from build123d import *

# Parameters (mm, degrees)
SKETCH_1_W          = 6
SKETCH_1_H          = 4
EXTRUDE_1_DEPTH     = 2
EXTRUDE_2_DEPTH     = 2
EXTRUDE_3_DEPTH     = 2
CUT_EXTRUDE_1_DEPTH = 2
CUT_EXTRUDE_2_DEPTH = 2


with BuildPart() as part:
    # 草圖1 → 填料-伸長1 (new body)
    with BuildSketch(Plane(origin=(0, 0, 0), x_dir=(1, 0, 0), z_dir=(0, 1, 0))):
        with Locations((3, 2)):
            Rectangle(SKETCH_1_W, SKETCH_1_H)
    extrude(amount=EXTRUDE_1_DEPTH)

    # 草圖2 → 填料-伸長2 (add)
    with BuildSketch(Plane(origin=(0, 2, 0), x_dir=(1, 0, 0), z_dir=(0, 1, 0))):
        Polygon((0, 4), (6, 2), (6, 4), align=None)
    extrude(amount=EXTRUDE_2_DEPTH)

    # 草圖4 → 填料-伸長3 (add)
    with BuildSketch(Plane(origin=(0, 2, 0), x_dir=(1, 0, 0), z_dir=(0, 1, 0))):
        Polygon((0, 0), (0, 2), (6, 0), align=None)
    extrude(amount=EXTRUDE_3_DEPTH)

    # Sketch 3D_1 → 除料-伸長1 (cut, along a direction that is not the sketch's normal)
    with BuildSketch(Plane(origin=(6, 2, -4), x_dir=(-0.9486832980505139, 0.316227766016838, 0), z_dir=(0.2294157338705617, 0.6882472016116854, -0.6882472016116854))):
        Polygon((0, 0), (0.632455532, 2.75680975), (6.32455532, 0), align=None)
    extrude(amount=CUT_EXTRUDE_1_DEPTH, dir=(0, 1, 0), mode=Mode.SUBTRACT)

    # Sketch 3D_2 → 除料-伸長2 (cut, along a direction that is not the sketch's normal)
    with BuildSketch(Plane(origin=(0, 2, 0), x_dir=(0.9486832980505139, 0.316227766016838, 0), z_dir=(-0.22941573387056177, 0.6882472016116853, 0.6882472016116854))):
        Polygon((0, 0), (0.632455532, 2.75680975), (6.32455532, 0), align=None)
    extrude(amount=CUT_EXTRUDE_2_DEPTH, dir=(0, 0, 1), mode=Mode.SUBTRACT)


solid = part.part
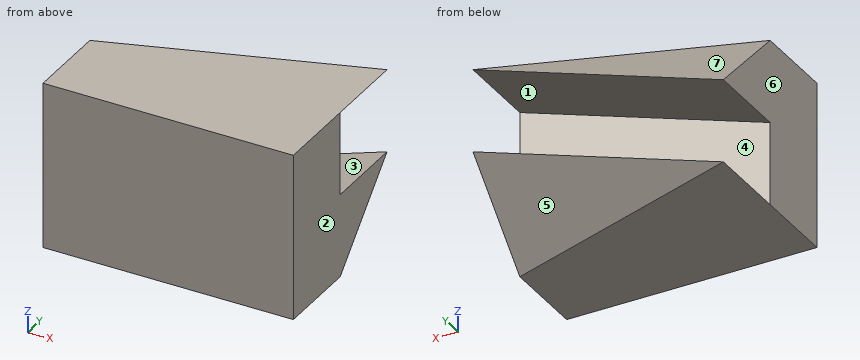
For this review, take the finished solid that the model builds, in its own axes (mm). Face numbers are marked on the shaded views. A direction names the side the tool comes from. Give positions to 0.01 mm unless a question says otherwise; leave off trailing zeros. Loops run counter-clockwise (first coordinate to the right, second up) from the corner with the lowest first, then second, coordinate; pieces in that order, holes last.
Item 1: For line 1 along Y through (x, z) = (4, -2.3); line 2 along Z through (x, y) = (5, 3.6); line 3 along Z through (x, y) = (3.75, 2.95), list the stretches that pass through material, from the lowest coordinate up.
Item 2: Take a section at C-C, the plane y = 3.4. State the section outline as (x, z) points.
Item 3: Take a section at A-A, the plane y = 2.35. State the section outline as (x, z) points.
Item 4: Take a section at B-B, the plane z = -1.2. State the section outline as (x, y) points, and give its area (3 significant figures).
Item 5: Tool access review of the marked faces 1, 2 and 3: name each direction out of +Z, -Z, +X, -X, +Y, -Y from which nothing blocks a thin tool from reaching the whole face with its end or side.
Item 6: Take a section at D-D, the plane x = 1.75. State the section outline as (y, z) points, and give its area (3 significant figures).
Item 7: Draft analysis for pull direction Z (two halves, no side actions). For the marked faces 4, 5, 6 and 7, state which applies: +Z half, -Z half, draft (parallel to the pull), parting line (faces both ways), or undercut.
Calculated:
1. line 1: y = 0 to 2
1. line 2: z = -2.73 to -2.33, -0.33 to 0
1. line 3: z = -3.8 to -2.75, -0.75 to 0
2. outline: (0, -4) - (1.8, -4) - (6, -2.6) - (6, -2) - close; (0, -2) - (6, 0) - (4.2, 0) - (0, -1.4) - close
3. outline: (0, -4) - (4.95, -4) - (6, -3.65) - (6, -2) - close; (0, -2) - (6, 0) - (1.05, 0) - (0, -0.35) - close
4. outline: (0, 0) - (6, 0) - (6, 2) - (2.4, 2) - (2.4, 4) - (0, 3.2) - close
4. area: 15.8 mm2
5. face 1: +X, +Y
5. face 2: +Z, -Z, +X, +Y, -Y
5. face 3: -X, +Y
6. outline: (0, -4) - (3.42, -4) - (4, -3.42) - (2, -3.42) - (2, -1.42) - (4, -1.42) - (2.58, 0) - (0, 0) - close
6. area: 10.8 mm2
7. face 4: undercut
7. face 5: -Z half
7. face 6: draft
7. face 7: +Z half
